Part model, mm, in its own coordinate system. Coordinates: 2 decimals unless noted, no trailing zeros. Loops run counter-clockwise (first coordinate to the right, second up) from the corner with the lowest first, then second, coordinate; pieces in that order, holes last. Notation, with made-up numbers: M 27.5,-33.5 L 41.5,-33.5 A33 ccw 41.5,1.5 Z; hole C 28.5,66.5 d11. An arc over 180 degrees is marked long. Answer as a JSON object with one key per item and string values. Group by question number.
1. Saw through at A-A on x = 30.75. Write the cut outline in (y, z).
2. Drop a flat-ended pin along its axis: pin 1 Ø4 at (x, y) = (9.25, -30.75) entering from +Z. Give the stop position or say it passes through.
3. Saw through at C-C on z = 1.75. Count the separate pieces of the cut face and the enclosed holes in it, then the cut area to 3 significant figures.
4. Mould opens along Y. For faces 1 (the face through (-1, -40, 3)), 2 (the face through (40, -1, 3)), 3 (the face through (-30.945, 32.237, 3.131)), 4 (the face through (-31.86, 21.01, 3.13)) say: released by +Y, released by -Y, zero draft, split by the parting line, or undercut.
from build123d import *

# Parameters (mm, degrees)
F0_R     = 1.5
F1_DEPTH = 6.35


with BuildPart() as f1:
    # F0 (on Top) → F1 (new body)
    with BuildSketch(Plane.XY):
        Polygon((0, 0), (9.25, 0), (40, 0), (40, 39.999997), (0, 39.999997), align=None)
        with Locations((9.25, 9.249999)):
            Circle(F0_R, mode=Mode.SUBTRACT)
        with Locations((20, 9.249999)):
            Circle(F0_R, mode=Mode.SUBTRACT)
        with Locations((30.75, 9.249999)):
            Circle(F0_R, mode=Mode.SUBTRACT)
        with Locations((9.25, 19.999998)):
            Circle(F0_R, mode=Mode.SUBTRACT)
        with Locations((9.25, 30.749998)):
            Circle(F0_R, mode=Mode.SUBTRACT)
        with Locations((20, 19.999998)):
            Circle(F0_R, mode=Mode.SUBTRACT)
        with Locations((30.75, 19.999998)):
            Circle(F0_R, mode=Mode.SUBTRACT)
        with Locations((20, 30.749998)):
            Circle(F0_R, mode=Mode.SUBTRACT)
        with Locations((30.75, 30.749998)):
            Circle(F0_R, mode=Mode.SUBTRACT)
        Polygon((40, 0), (9.25, 0), (0, 0), (0, -39.999997), (40, -39.999997), align=None)
        with Locations((9.25, -30.749998)):
            Circle(F0_R, mode=Mode.SUBTRACT)
        with Locations((9.25, -19.999998)):
            Circle(F0_R, mode=Mode.SUBTRACT)
        with Locations((20, -30.749998)):
            Circle(F0_R, mode=Mode.SUBTRACT)
        with Locations((30.75, -30.749998)):
            Circle(F0_R, mode=Mode.SUBTRACT)
        with Locations((20, -19.999998)):
            Circle(F0_R, mode=Mode.SUBTRACT)
        with Locations((30.75, -19.999998)):
            Circle(F0_R, mode=Mode.SUBTRACT)
        with Locations((9.25, -9.249999)):
            Circle(F0_R, mode=Mode.SUBTRACT)
        with Locations((20, -9.249999)):
            Circle(F0_R, mode=Mode.SUBTRACT)
        with Locations((30.75, -9.249999)):
            Circle(F0_R, mode=Mode.SUBTRACT)
        Polygon((0, -39.999997), (0, 0), (0, 39.999997), (-40, 39.999997), (-40, 0), (-40, -39.999997), align=None)
        with Locations((-30.75, -30.749998)):
            Circle(F0_R, mode=Mode.SUBTRACT)
        with Locations((-30.75, -19.999998)):
            Circle(F0_R, mode=Mode.SUBTRACT)
        with Locations((-20, -30.749998)):
            Circle(F0_R, mode=Mode.SUBTRACT)
        with Locations((-9.25, -30.749998)):
            Circle(F0_R, mode=Mode.SUBTRACT)
        with Locations((-20, -19.999998)):
            Circle(F0_R, mode=Mode.SUBTRACT)
        with Locations((-9.25, -19.999998)):
            Circle(F0_R, mode=Mode.SUBTRACT)
        with Locations((-30.75, -9.249999)):
            Circle(F0_R, mode=Mode.SUBTRACT)
        with Locations((-20, -9.249999)):
            Circle(F0_R, mode=Mode.SUBTRACT)
        with Locations((-9.25, -9.249999)):
            Circle(F0_R, mode=Mode.SUBTRACT)
        with Locations((-30.75, 9.249999)):
            Circle(F0_R, mode=Mode.SUBTRACT)
        with Locations((-20, 9.249999)):
            Circle(F0_R, mode=Mode.SUBTRACT)
        with Locations((-9.25, 9.249999)):
            Circle(F0_R, mode=Mode.SUBTRACT)
        with Locations((-30.75, 19.999998)):
            Circle(F0_R, mode=Mode.SUBTRACT)
        with Locations((-30.75, 30.749998)):
            Circle(F0_R, mode=Mode.SUBTRACT)
        with Locations((-20, 19.999998)):
            Circle(F0_R, mode=Mode.SUBTRACT)
        with Locations((-9.25, 19.999998)):
            Circle(F0_R, mode=Mode.SUBTRACT)
        with Locations((-20, 30.749998)):
            Circle(F0_R, mode=Mode.SUBTRACT)
        with Locations((-9.25, 30.749998)):
            Circle(F0_R, mode=Mode.SUBTRACT)
    extrude(amount=F1_DEPTH)


solid = f1.part
Outcome:
{
 "1": {"outline": "M -40,0 L -32.25,0 L -32.25,6.35 L -40,6.35 Z; M -29.25,0 L -21.5,0 L -21.5,6.35 L -29.25,6.35 Z; M -18.5,0 L -10.75,0 L -10.75,6.35 L -18.5,6.35 Z; M -7.75,0 L 7.75,0 L 7.75,6.35 L -7.75,6.35 Z; M 10.75,0 L 18.5,0 L 18.5,6.35 L 10.75,6.35 Z; M 21.5,0 L 29.25,0 L 29.25,6.35 L 21.5,6.35 Z; M 32.25,0 L 40,0 L 40,6.35 L 32.25,6.35 Z"},
 "2": {"pin 1": "stops at z = 6.35"},
 "3": {"separate pieces": "1", "enclosed holes": "36", "area": "6,150 mm²"},
 "4": {"face 1": "released by -Y", "face 2": "zero draft", "face 3": "undercut", "face 4": "undercut"}
}
